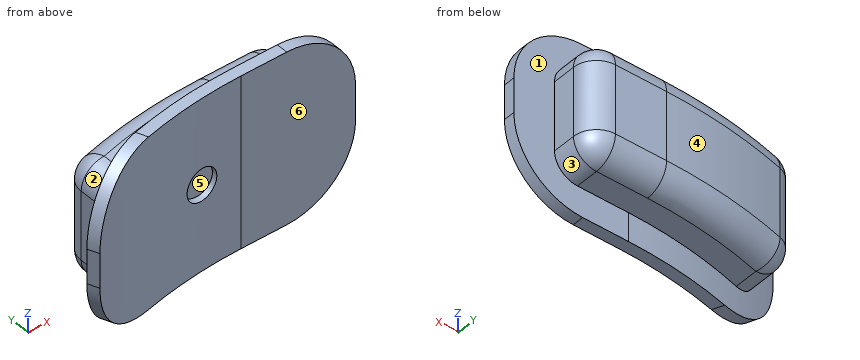
from build123d import *

# Parameters (mm, degrees)
BOSS_EXTRUDE3_DEPTH                  = 19.05
SKETCH5_R                            = 1.778
CUT_EXTRUDE1_DEPTH                   = 3.048
SKETCH7_W                            = 24.13
SKETCH7_H                            = 12.7
BOSS_EXTRUDE4_DEPTH                  = 6.35
BOSS_EXTRUDE4_DIRECTION_2_REACH      = 29.38
BOSS_EXTRUDE4_DIRECTION_2_END_RADIUS = 50.8
CUT_EXTRUDE2_DEPTH                   = 26.597668413
FILLET1_R                            = 2.54
FILLET2_R                            = 7.62


with BuildPart() as part:
    # Sketch3 → Boss-Extrude3 (new body)
    with BuildSketch(Plane.XY):
        with BuildLine():
            Line((0, 0), (12.7, 0))
            Line((12.7, 0), (12.7, -1.27))
            Line((12.7, -1.27), (0, -1.27))
            ThreePointArc((0, -1.27), (-9.461085009, -2.182011863), (-18.57375, -4.884461117))
            Line((-18.57375, -4.884461117), (-19.05, -3.707139607))
            ThreePointArc((-19.05, -3.707139607), (-9.703676933, -0.935396783), (0, 0))
        make_face()
    extrude(amount=BOSS_EXTRUDE3_DEPTH)

    # Sketch5 → Cut-Extrude1 (cut)
    with BuildSketch(Plane(origin=(0, -3.81, 0), x_dir=(-1, 0, 0), z_dir=(0, -1, 0))):
        with Locations(Location((4.49834, -9.525, 0), (0, 0, 90))):
            Circle(SKETCH5_R)
    extrude(amount=-CUT_EXTRUDE1_DEPTH, mode=Mode.SUBTRACT)

    # Sketch7 → Boss-Extrude4 (add)
    with BuildSketch(Plane(origin=(0, 0, 0), x_dir=(1, 0, 0), z_dir=(0, 1, 0))):
        with Locations((-3.86334, -9.525)):
            Rectangle(SKETCH7_W, SKETCH7_H)
    extrude(amount=BOSS_EXTRUDE4_DEPTH)

    # Boss-Extrude4 direction 2: up to this cylinder (the profile starts outside it)
    boss_extrude4_direction_2_end = Plane(origin=(0, -50.8, 9.525), z_dir=(0, 0, -1)) * Cylinder(BOSS_EXTRUDE4_DIRECTION_2_END_RADIUS, 161.36, mode=Mode.PRIVATE)
    # Sketch7 → Boss-Extrude4 direction 2 (add, up to the surface)
    with BuildSketch(Plane(origin=(0, 0, 0), x_dir=(1, 0, 0), z_dir=(0, 1, 0)), mode=Mode.PRIVATE) as boss_extrude4_direction_2_sk1:
        with Locations((-3.86334, -9.525)):
            Rectangle(SKETCH7_W, SKETCH7_H)
    boss_extrude4_direction_2_tool1 = extrude(boss_extrude4_direction_2_sk1.sketch, amount=-BOSS_EXTRUDE4_DIRECTION_2_REACH, mode=Mode.PRIVATE) - boss_extrude4_direction_2_end
    add(boss_extrude4_direction_2_tool1.solids().sort_by_distance((-3.86334, 0, 9.525))[0])
    add(boss_extrude4_direction_2_tool1.solids().sort_by_distance((-3.86334, 0, 9.525))[1])

    # Sketch8 → Cut-Extrude2 (cut, through all)
    with BuildSketch(Plane.XY.offset(15.875)):
        with BuildLine():
            Line((8.20166, 5.08), (8.20166, 6.35))
            Line((8.20166, 6.35), (-20.955, 6.35))
            Line((-20.955, 6.35), (-20.955, 1.002146432))
            ThreePointArc((-20.955, 1.002146432), (-10.674044626, 4.051063539), (0, 5.08))
            Line((0, 5.08), (8.20166, 5.08))
        make_face()
    extrude(amount=-CUT_EXTRUDE2_DEPTH, mode=Mode.SUBTRACT)

    # Fillet1
    fillet1_edges = [part.edges().sort_by_distance(p)[0] for p in [
        (-15.92834, 0.100002136, 3.175),
        (-15.92834, 0.100002136, 15.875),
        (8.20166, 2.54, 3.175),
        (8.20166, 2.54, 15.875),
        (-15.92834, 2.761762339, 9.525),
        (-8.048078047, 4.497403553, 3.175),
        (4.10083, 5.08, 3.175),
        (8.20166, 5.08, 9.525),
        (-8.048078047, 4.497403553, 15.875),
        (4.10083, 5.08, 15.875),
    ]]
    fillet(fillet1_edges, radius=FILLET1_R)

    # Fillet2
    fillet2_edges = [part.edges().sort_by_distance(p)[0] for p in [
        (-18.811875, -4.295800362, 19.05),
        (-18.811875, -4.295800362, 0),
        (12.7, -0.635, 19.05),
        (12.7, -0.635, 0),
    ]]
    fillet(fillet2_edges, radius=FILLET2_R)


solid = part.part
Could you check a few things on this model? Use its own coordinates, in mm. Face numbers are marked on the shaded views. A direction names the side the tool comes from. Give positions to 0.01 mm unless a question says otherwise; leave off trailing zeros. Write each loop counter-clockwise with the first axis right and the second up, starting at its lowest first coordinate (ties: lowest second). Pieces come first, ordered by that corner, then holes. Notation, with made-up numbers: (-28.5, -15) - (-22.5, -15) arc R18 cw to (-22.5, -3) - close; hole circle Ø1 at (55, 19.5). An arc over 180 degrees is marked (long way). Use CSV: the item, a comma, the result in double quotes. Start each with the question number.
Item 1: If we mould it in two halves opening along X, with no side actions, what happens to the marked faces 4, 5 and 6? For each: pulls with the +X half, pulls with the -X half, needs draft (parallel to the pull), parting line crosses it, or undercut.
Item 2: I want a section at D-D, the plane x = 10. Please give me the cut outline in (y, z).
Item 3: I'm going to push flat-ended pins straight in: pin 1 (2 mm diameter, centred on y = 3.5, z = 6.5, fed in from +X); pin 2 (5 mm diameter, centred on x = -7.5, y = 4, fed in from +Z) (3 decimals); pin 3 (1 mm diameter, centred on x = -1.5, z = 5, fed in from +Y). Where does each tip first touch, or does it pass through?
Item 4: If I drill on line 1 along Y through (x, z) = (9, 10); line 2 along Z through (x, y) = (-11.5, 0.75) (3 decimals); line 3 along Y through (x, z) = (5.5, 9), over which ranges is the centre line in solid material (lowest first)?
Item 5: I want a section at A-A, the plane x = 3. Please give me the cut outline in (y, z) (3 decimals), then the cut area to 3 significant figures.
Item 6: For the marked faces 1, 2 and 3, which set-ups out of +Z, -Z, +X, -X, +Y, -Y let a thin tool reach every point of the face, with its end or its side?
Item 7: I want a section at B-B, the plane z = 10.5. Please give me the cut outline in (x, y).
Item 8: I want a section at C-C, the plane z = 4.5. Please give me the cut outline in (x, y).
Findings:
1,face 4,"pulls with the -X half"
1,face 5,"undercut"
1,face 6,"needs draft"
2,outline,"(-1.27, 1.8) - (0, 1.8) - (0, 17.25) - (-1.27, 17.25) - close"
3,pin 1,"stops at x = 8.2"
3,pin 2,"stops at z = 15.875"
3,pin 3,"stops at y = 5.05"
4,line 1,"y = -1.27 to 0"
4,line 2,"z = 3.175 to 15.875"
4,line 3,"y = -1.27 to 5.08"
5,outline,"(-1.27, 0) - (0, 0) - (0, 3.175) - (2.54, 3.175) arc R2.54 ccw to (5.08, 5.715) - (5.08, 13.335) arc R2.54 ccw to (2.54, 15.875) - (0, 15.875) - (0, 19.05) - (-1.27, 19.05) - close"
5,area,"85.9 mm2"
6,face 1,"+X, +Y"
6,face 2,"+Z, -X, +Y"
6,face 3,"-Z, +X, +Y"
7,outline,"(-19.05, -3.71) - (-18.57, -4.88) arc R49.53 cw to (-5.99, -1.63) - (-5.99, -0.76) - (-3.01, -0.76) - (-3.01, -1.36) arc R49.53 cw to (0, -1.27) - (12.7, -1.27) - (12.7, 0) - (8.2, 0) - (8.2, 2.54) arc R2.54 ccw to (5.66, 5.08) - (0, 5.08) arc R55.88 ccw to (-14.03, 3.29) arc R2.54 ccw to (-15.93, 0.83) - (-15.93, -2.56) arc R50.8 ccw to start"
8,outline,"(-18.43, -3.46) - (-17.95, -4.64) arc R49.53 cw to (0, -1.27) - (12.03, -1.27) - (12.03, 0) - (7.89, 0) - (7.89, 2.54) arc R2.23 ccw to (5.66, 4.77) - (0, 4.77) arc R55.57 ccw to (-13.95, 2.99) arc R2.23 ccw to (-15.62, 0.83) - (-15.62, -2.46) arc R50.8 ccw to start"
